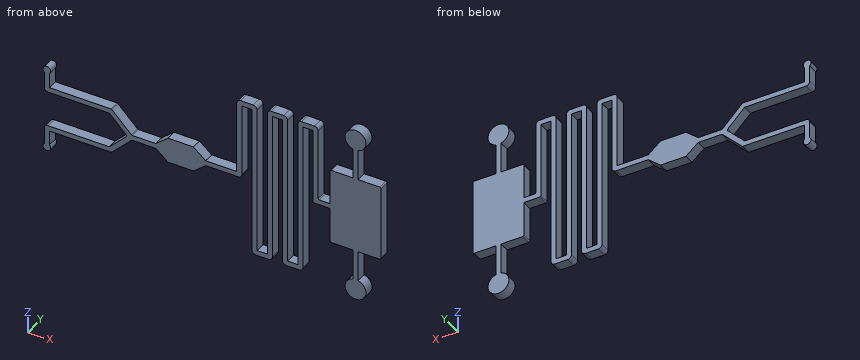
from build123d import *

# Parameters (mm, degrees)
BOSS_EXTRUDE1_DEPTH = 2


with BuildPart() as part:
    # Sketch2 → Boss-Extrude1 (new body)
    with BuildSketch(Plane(origin=(0, 0, 0), x_dir=(1, 0, 0), z_dir=(0, 1, 0))):
        with BuildLine():
            Line((15.163755459, 7.25), (15.163755459, -7.25))
            ThreePointArc((15.163755459, -7.25), (15.090532154, -7.426776695), (14.913755459, -7.5))
            Line((14.913755459, -7.5), (10.663755459, -7.5))
            Line((10.663755459, -7.5), (10.663755459, -13.511910465))
            ThreePointArc((10.663755459, -13.511910465), (10.163755459, -17.55), (9.663755459, -13.511910465))
            Line((9.663755459, -13.511910465), (9.663755459, -7.5))
            Line((9.663755459, -7.5), (5.413755459, -7.5))
            ThreePointArc((5.413755459, -7.5), (5.236978763, -7.426776695), (5.163755459, -7.25))
            Line((5.163755459, -7.25), (5.163755459, -0.5))
            Line((5.163755459, -0.5), (3.075114856, -0.5))
            ThreePointArc((3.075114856, -0.5), (2.898338161, -0.573223305), (2.825114856, -0.75))
            Line((2.825114856, -0.75), (2.825114856, -14.75))
            ThreePointArc((2.825114856, -14.75), (2.605444942, -15.280330086), (2.075114856, -15.5))
            Line((2.075114856, -15.5), (-0.424885144, -15.5))
            ThreePointArc((-0.424885144, -15.5), (-0.95521523, -15.280330086), (-1.174885144, -14.75))
            Line((-1.174885144, -14.75), (-1.174885144, 14.5))
            Line((-1.174885144, 14.5), (-3.174885144, 14.5))
            Line((-3.174885144, 14.5), (-3.174885144, -14.75))
            ThreePointArc((-3.174885144, -14.75), (-3.394555058, -15.280330086), (-3.924885144, -15.5))
            Line((-3.924885144, -15.5), (-6.424885144, -15.5))
            ThreePointArc((-6.424885144, -15.5), (-6.95521523, -15.280330086), (-7.174885144, -14.75))
            Line((-7.174885144, -14.75), (-7.174885144, 14.5))
            Line((-7.174885144, 14.5), (-9.174885144, 14.5))
            Line((-9.174885144, 14.5), (-9.174885144, -14.75))
            ThreePointArc((-9.174885144, -14.75), (-9.394555058, -15.280330086), (-9.924885144, -15.5))
            Line((-9.924885144, -15.5), (-12.424885144, -15.5))
            ThreePointArc((-12.424885144, -15.5), (-12.95521523, -15.280330086), (-13.174885144, -14.75))
            Line((-13.174885144, -14.75), (-13.174885144, -0.5))
            Line((-13.174885144, -0.5), (-19.274885144, -0.5))
            Line((-19.274885144, -0.5), (-21.674885144, -2.5))
            Line((-21.674885144, -2.5), (-26.674885144, -2.5))
            Line((-26.674885144, -2.5), (-29.074885144, -0.5))
            Line((-29.074885144, -0.5), (-33.68175141, -0.5))
            ThreePointArc((-33.68175141, -0.5), (-33.777422268, -0.519030117), (-33.858528105, -0.573223305))
            Line((-33.858528105, -0.573223305), (-37.712081496, -4.426776695))
            ThreePointArc((-37.712081496, -4.426776695), (-37.793187333, -4.480969883), (-37.888858191, -4.5))
            Line((-37.888858191, -4.5), (-46.992411582, -4.5))
            Line((-46.992411582, -4.5), (-49.992411582, -4.5))
            Line((-49.992411582, -4.5), (-49.992411582, -7.440983006))
            ThreePointArc((-49.992411582, -7.440983006), (-50.492411582, -8.75), (-50.992411582, -7.440983006))
            Line((-50.992411582, -7.440983006), (-50.992411582, -4.25))
            ThreePointArc((-50.992411582, -4.25), (-50.772741668, -3.719669914), (-50.242411582, -3.5))
            Line((-50.242411582, -3.5), (-38.303071753, -3.5))
            ThreePointArc((-38.303071753, -3.5), (-38.207400895, -3.480969883), (-38.126295058, -3.426776695))
            Line((-38.126295058, -3.426776695), (-34.876295058, -0.176776695))
            ThreePointArc((-34.876295058, -0.176776695), (-34.803071753, 0), (-34.876295058, 0.176776695))
            Line((-34.876295058, 0.176776695), (-38.126295058, 3.426776695))
            ThreePointArc((-38.126295058, 3.426776695), (-38.207400895, 3.480969883), (-38.303071753, 3.5))
            Line((-38.303071753, 3.5), (-46.242411582, 3.5))
            Line((-46.242411582, 3.5), (-50.242411582, 3.5))
            ThreePointArc((-50.242411582, 3.5), (-50.772741668, 3.719669914), (-50.992411582, 4.25))
            Line((-50.992411582, 4.25), (-50.992411582, 7.440983006))
            ThreePointArc((-50.992411582, 7.440983006), (-50.492411582, 8.75), (-49.992411582, 7.440983006))
            Line((-49.992411582, 7.440983006), (-49.992411582, 4.5))
            Line((-49.992411582, 4.5), (-46.992411582, 4.5))
            Line((-46.992411582, 4.5), (-37.888858191, 4.5))
            ThreePointArc((-37.888858191, 4.5), (-37.793187333, 4.480969883), (-37.712081496, 4.426776695))
            Line((-37.712081496, 4.426776695), (-33.858528105, 0.573223305))
            ThreePointArc((-33.858528105, 0.573223305), (-33.777422268, 0.519030117), (-33.68175141, 0.5))
            Line((-33.68175141, 0.5), (-29.074885144, 0.5))
            Line((-29.074885144, 0.5), (-26.674885144, 2.5))
            Line((-26.674885144, 2.5), (-21.674885144, 2.5))
            Line((-21.674885144, 2.5), (-19.274885144, 0.5))
            Line((-19.274885144, 0.5), (-12.924885144, 0.5))
            ThreePointArc((-12.924885144, 0.5), (-12.394555058, 0.280330086), (-12.174885144, -0.25))
            Line((-12.174885144, -0.25), (-12.174885144, -14.5))
            Line((-12.174885144, -14.5), (-10.174885144, -14.5))
            Line((-10.174885144, -14.5), (-10.174885144, 14.75))
            ThreePointArc((-10.174885144, 14.75), (-9.95521523, 15.280330086), (-9.424885144, 15.5))
            Line((-9.424885144, 15.5), (-6.924885144, 15.5))
            ThreePointArc((-6.924885144, 15.5), (-6.394555058, 15.280330086), (-6.174885144, 14.75))
            Line((-6.174885144, 14.75), (-6.174885144, -14.5))
            Line((-6.174885144, -14.5), (-4.174885144, -14.5))
            Line((-4.174885144, -14.5), (-4.174885144, 14.75))
            ThreePointArc((-4.174885144, 14.75), (-3.95521523, 15.280330086), (-3.424885144, 15.5))
            Line((-3.424885144, 15.5), (-0.924885144, 15.5))
            ThreePointArc((-0.924885144, 15.5), (-0.394555058, 15.280330086), (-0.174885144, 14.75))
            Line((-0.174885144, 14.75), (-0.174885144, -14.5))
            Line((-0.174885144, -14.5), (1.825114856, -14.5))
            Line((1.825114856, -14.5), (1.825114856, 0.25))
            ThreePointArc((1.825114856, 0.25), (1.898338161, 0.426776695), (2.075114856, 0.5))
            Line((2.075114856, 0.5), (5.163755459, 0.5))
            Line((5.163755459, 0.5), (5.163755459, 7.25))
            ThreePointArc((5.163755459, 7.25), (5.236978763, 7.426776695), (5.413755459, 7.5))
            Line((5.413755459, 7.5), (9.663755459, 7.5))
            Line((9.663755459, 7.5), (9.663755459, 13.511910465))
            ThreePointArc((9.663755459, 13.511910465), (10.163755459, 17.55), (10.663755459, 13.511910465))
            Line((10.663755459, 13.511910465), (10.663755459, 7.5))
            Line((10.663755459, 7.5), (14.913755459, 7.5))
            ThreePointArc((14.913755459, 7.5), (15.090532154, 7.426776695), (15.163755459, 7.25))
        make_face()
    extrude(amount=BOSS_EXTRUDE1_DEPTH)


solid = part.part
Read the model definition and answer for the solid it produces. Units are mm, in the model's axes. Give positions to 0.01 mm unless a question says otherwise; leave off trailing zeros. Loops run counter-clockwise (first coordinate to the right, second up) from the corner with the lowest first, then second, coordinate; pieces in that order, holes last. Notation, with made-up numbers: M -33.5,52 L -4.5,52 A33 ccw -4.5,88 Z; hole C 16.5,0 d10. An arc over 180 degrees is marked long. Write each question's results on one line, items separated by ' | '.
1. Section C-C on x = -24.5 is taken. Give the vertices of the cut face in (y, z).
Values:
outline: M 0,-2.5 L 2,-2.5 L 2,2.5 L 0,2.5 Z
2. Section B-B on x = -41 is taken. Give the vertices of the cut face in (y, z), plus the area to 3 significant figures.
Values:
outline: M 0,-4.5 L 2,-4.5 L 2,-3.5 L 0,-3.5 Z; M 0,3.5 L 2,3.5 L 2,4.5 L 0,4.5 Z | area: 4.00 mm^2
3. Section D-D on x = -2.5 is taken. Give the vertices of the cut face in (y, z), plus the area to 3 significant figures.
Values:
outline: M 0,-15.5 L 2,-15.5 L 2,-14.5 L 0,-14.5 Z | area: 2.00 mm^2
4. Given pin 1 (1 mm diameter, centred on y = 1, z = 4.5, fed in from -X); pin 2 (1 mm diameter, centred on x = 0.5, y = 1.5, fed in from +Z); pin 3 (1 mm diameter, centred on x = -45.5, y = 0.5, fed in from +Z), each flat-ended and moving along its own axis, determine where each tip first touches the part or whether it passes through.
Values:
pin 1: stops at x = -50.99 | pin 2: stops at z = 15.5 | pin 3: stops at z = 4.5
5. Straight lines are drawn through the part: line 1 (X direction, y = 1.4, z = -12); line 2 (Z direction, x = -46, y = 1.55); line 3 (X direction, y = 0.85, z = -8.5). For each, find the intervals that lie inside material, in ascending order. Write a range as [from, to].
Values:
line 1: x = [-10.17, -9.17], [-7.17, -6.17], [-4.17, -3.17], [-1.17, -0.17], [9.66, 10.66] | line 2: z = [-4.5, -3.5], [3.5, 4.5] | line 3: x = [-51.05, -49.93], [-10.17, -9.17], [-7.17, -6.17], [-4.17, -3.17], [-1.17, -0.17], [9.66, 10.66]
6. Section A-A on z = 12.5 is taken. Give the vertices of the cut face in (x, y), plus the area to 3 significant figures.
Values:
outline: M -13.17,0 L -12.17,0 L -12.17,2 L -13.17,2 Z; M -10.17,0 L -9.17,0 L -9.17,2 L -10.17,2 Z; M -7.17,0 L -6.17,0 L -6.17,2 L -7.17,2 Z; M -4.17,0 L -3.17,0 L -3.17,2 L -4.17,2 Z; M -1.17,0 L -0.17,0 L -0.17,2 L -1.17,2 Z; M 1.83,0 L 2.83,0 L 2.83,2 L 1.83,2 Z; M 9.66,0 L 10.66,0 L 10.66,2 L 9.66,2 Z | area: 14.0 mm^2
